Read the model definition and answer for the solid it produces. Units are mm, in the model's axes. Coordinates: 2 decimals unless noted, no trailing zeros. Write each loop counter-clockwise with the first axis right and the second up, starting at its lowest first coordinate (ties: lowest second). Pieces come first, ordered by that corner, then holes.
Item 1: Section C-C (y = -10.75) is taken. Give the vertices of the cut face in (x, z) (3 decimals).
Item 2: Determine the mould class of faces 1 (the face through (19, -11, 12.7)), 2 (the face through (38.1, -9, 6)), 3 (the face through (3.355, -8.766, 6.693)) for opening direction Z: released by +Z, released by -Z, zero draft, split by the parting line, or undercut.
Item 3: Section A-A (z = 6.35) is taken. Give the vertices of the cut face in (x, y), then the cut area to 3 significant figures.
Item 4: Straight lines are drawn through the part: probe 1 along X at (y, z) = (-6, 12); probe 2 along X at (y, z) = (-2.75, 1.75); probe 3 along Z at (x, y) = (34.5, -14.75). For each, find the intervals that lie inside material, in ascending order.
Item 5: Each of these flat-tipped pins is pushed along its axis until it touches: P1, Ø2, axis at x = 17, y = -12.5, coming from the -Z side; P2, Ø2, axis at x = 33.655, z = 6.35, coming from the -Y side. Where does it stop, or does it pass through?
Item 6: Section B-B (y = -4.5) is taken. Give the vertices of the cut face in (x, z) (3 decimals), then the cut area to 3 significant figures.
Item 7: Section D-D (x = 19.05) is taken. Give the vertices of the cut face in (y, z).
from build123d import *

# Parameters (mm, degrees)
SKETCH1_W           = 38.1
SKETCH1_H           = 17.78
BOSS_EXTRUDE1_DEPTH = 12.7
CUT_EXTRUDE1_DEPTH  = 13.7
CUT_EXTRUDE2_DEPTH  = 18.78


with BuildPart() as part:
    # Sketch1 → Boss-Extrude1 (new body)
    with BuildSketch(Plane.XY):
        with Locations((19.05, -8.89)):
            Rectangle(SKETCH1_W, SKETCH1_H)
    extrude(amount=BOSS_EXTRUDE1_DEPTH)

    # Sketch4 → Cut-Extrude1 (cut, through all)
    with BuildSketch(Plane.XY.offset(12.7)):
        with BuildLine():
            Line((19.05, 0), (29.21, 0))
            ThreePointArc((29.21, 0), (19.05, -10.16), (8.89, 0))
            Line((8.89, 0), (19.05, 0))
        make_face()
    extrude(amount=-CUT_EXTRUDE1_DEPTH, mode=Mode.SUBTRACT)

    # Sketch5 → Cut-Extrude2 (cut, through all)
    with BuildSketch(Plane(origin=(0, 0, 0), x_dir=(1, 0, 0), z_dir=(0, 1, 0))):
        with BuildLine():
            ThreePointArc((5.588, -6.35), (4.445, -5.207), (3.302, -6.35))
            Line((3.302, -6.35), (5.588, -6.35))
        make_face()
        with BuildLine():
            Line((5.588, -6.35), (3.302, -6.35))
            ThreePointArc((3.302, -6.35), (4.445, -7.493), (5.588, -6.35))
        make_face()
        with BuildLine():
            ThreePointArc((32.512, -6.35), (33.655, -7.493), (34.798, -6.35))
            Line((34.798, -6.35), (32.512, -6.35))
        make_face()
        with BuildLine():
            Line((32.512, -6.35), (34.798, -6.35))
            ThreePointArc((34.798, -6.35), (33.655, -5.207), (32.512, -6.35))
        make_face()
    extrude(amount=-CUT_EXTRUDE2_DEPTH, mode=Mode.SUBTRACT)


solid = part.part
Established:
1. outline: (0, 0) - (38.1, 0) - (38.1, 12.7) - (0, 12.7) - close; hole circle Ø2.286 at (4.445, 6.35); hole circle Ø2.286 at (33.655, 6.35)
2. face 1: released by +Z
2. face 2: zero draft
2. face 3: undercut
3. outline: (0, -17.78) - (3.3, -17.78) - (3.3, 0) - (0, 0) - close; (5.59, -17.78) - (32.51, -17.78) - (32.51, 0) - (29.21, 0) arc R10.16 cw to (8.89, 0) - (5.59, 0) - close; (34.8, -17.78) - (38.1, -17.78) - (38.1, 0) - (34.8, 0) - close
3. area: 434 mm2
4. probe 1: x = 0 to 10.85, 27.25 to 38.1
4. probe 2: x = 0 to 9.27, 28.83 to 38.1
4. probe 3: z = 0 to 5.58, 7.12 to 12.7
5. P1: stops at z = 0
5. P2: passes through
6. outline: (0, 0) - (9.941, 0) - (9.941, 12.7) - (0, 12.7) - close; (28.159, 0) - (38.1, 0) - (38.1, 12.7) - (28.159, 12.7) - close; hole circle Ø2.286 at (4.445, 6.35); hole circle Ø2.286 at (33.655, 6.35)
6. area: 244 mm2
7. outline: (-17.78, 0) - (-10.16, 0) - (-10.16, 12.7) - (-17.78, 12.7) - close
